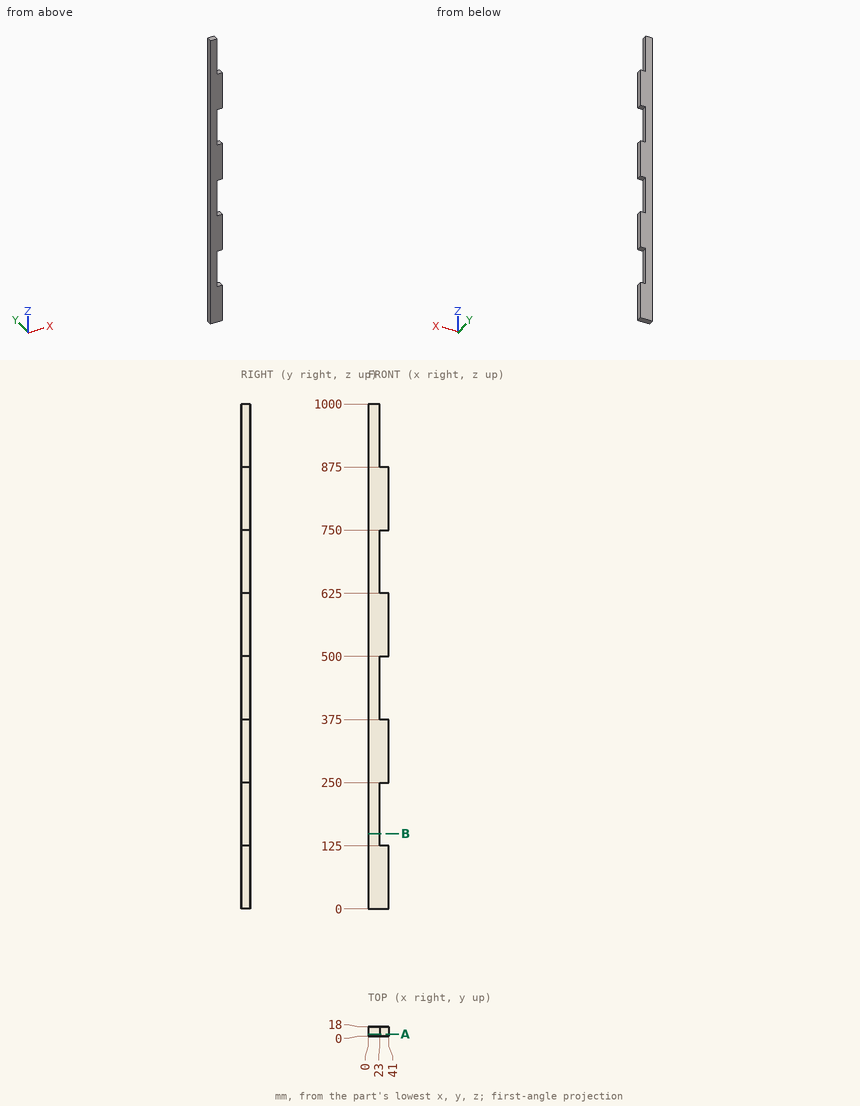
Answer from the drawing. Dimensions are ordinates in mm from the lowest x, y and z of the part. Coordinates: 2 decimals unless noted, no trailing zeros. Loops run counter-clockwise (first coordinate to the right, second up) from the corner with the lowest first, then second, coordinate; pieces in that order, holes last.
Q1. Consider probe 1 along Z at (x, y) = (33, 7.25); probe 2 along X at (y, z) = (7.5, 431). Determine where each line is inside the solid, lowest interval first.
Q2. Each of these flat-tipped pins is pushed along its axis until it touches: pin 1 Ø5 at (y, z) = (4.5, 633.5) entering from +X; pin 2 Ø5.5 at (x, y) = (34, 9) entering from +Z. Where does it stop, or does it pass through?
Q3. The part is cut by section B-B on z = 149. Write down the section's boundary in (x, y).
Q4. The part is cut by section A-A on y = 3.75. Write down the section's boundary in (x, z), and give its area (3 significant figures).
Results below:
1. probe 1: z = 0 to 125, 250 to 375, 500 to 625, 750 to 875
1. probe 2: x = 0 to 23
2. pin 1: stops at x = 23
2. pin 2: stops at z = 875
3. outline: (0, 0) - (23, 0) - (23, 18) - (0, 18) - close
4. outline: (0, 0) - (41, 0) - (41, 125) - (23, 125) - (23, 250) - (41, 250) - (41, 375) - (23, 375) - (23, 500) - (41, 500) - (41, 625) - (23, 625) - (23, 750) - (41, 750) - (41, 875) - (23, 875) - (23, 1000) - (0, 1000) - close
4. area: 32,000 mm2
